Can you work these out from the model? Positions are in its coordinate system, mm. Face numbers are marked on the shaded views. A direction names the side the tool comes from. Give positions to 0.01 mm unless a question says otherwise; leave off trailing zeros. Order: outer loops, then holes, each group sorted by start corner. A loop starts at its lowest first (then second) coordinate and runs counter-clockwise, first axis right, second up. Notation, with made-up numbers: (-8, 26.25) - (27, 26.25) arc R24 cw to (27, 44.25) - close; hole circle Ø6 at (8, 41). An arc over 180 degrees is marked (long way). One line per question, with ' | ' between items.
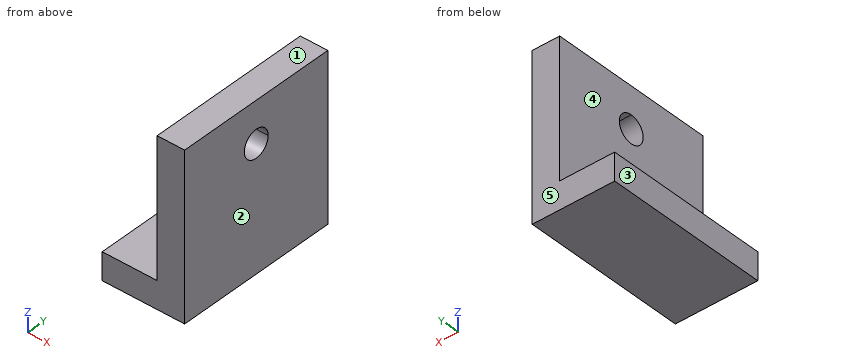
```python
from build123d import *

# Parameters (mm, degrees)
F1_DEPTH = 76.2
F3_DEPTH = 50.8


with BuildPart() as f1:
    # F0 (on Front) → F1 (new body, symmetric)
    with BuildSketch(Plane.XZ):
        Polygon((-76.2, 0), (0, 0), (0, 152.4), (-25.4, 152.4), (-25.4, 25.4), (-76.2, 25.4), align=None)
    extrude(amount=F1_DEPTH, both=True)

    # F2 (on face) → F3 (cut)
    with BuildSketch(Plane.YZ):
        with BuildLine():
            Line((0, 114.3), (0, 127))
            ThreePointArc((0, 127), (-8.980256, 105.319744), (12.7, 114.3))
            Line((12.7, 114.3), (0, 114.3))
        make_face()
        with BuildLine():
            ThreePointArc((12.7, 114.3), (8.980256, 123.280256), (0, 127))
            Line((0, 127), (0, 114.3))
            Line((0, 114.3), (12.7, 114.3))
        make_face()
    extrude(amount=-F3_DEPTH, mode=Mode.SUBTRACT)


solid = f1.part
```
(1) Imagine slicing it at B-B (y = -29). List the corners of the cut face in (x, z) for me, and give its area (3 significant figures).
Answer below:
outline: (-76.2, 0) - (0, 0) - (0, 152.4) - (-25.4, 152.4) - (-25.4, 25.4) - (-76.2, 25.4) - close | area: 5,160 mm^2
(2) On a 3-axis mill with a long thin cutter (end or side, diameter ignored), from which of +Z, -Z, +X, -X, +Y, -Y can I reach the whole of each face in a straight line? I mean the marked faces 4 and 5. Say none if no direction works.
Answer below:
face 4: +Z, -X, +Y, -Y | face 5: +Z, -Z, +X, -X, +Y
(3) Imagine slicing it at A-A (z = 106.5). List the corners of the cut face in (x, y) for me, and give its area (3 significant figures).
Answer below:
outline: (-25.4, -76.2) - (0, -76.2) - (0, -10.02) - (-25.4, -10.02) - close; (-25.4, 10.02) - (0, 10.02) - (0, 76.2) - (-25.4, 76.2) - close | area: 3,360 mm^2
(4) Imagine slicing it at D-D (z = 135.5). List the corners of the cut face in (x, y) for me.
Answer below:
outline: (-25.4, -76.2) - (0, -76.2) - (0, 76.2) - (-25.4, 76.2) - close
(5) Will this pin go through, and if not, where does the flat tip stop? pin 1 (10 mm diameter, centred on x = -45.5, y = -41.5, fed in from +Z).
Answer below:
pin 1: z = 25.4
(6) If we mould it in two halves opening along X, with no side actions, what happens to the marked faces 1, 2 and 3? For each: released by +X, released by -X, zero draft, split by the parting line, or undercut.
Answer below:
face 1: zero draft | face 2: released by +X | face 3: released by -X
(7) If I drill on line 1 (Y direction, x = -11.25, z = 114.3); line 2 (Z direction, x = -10.25, y = 0); line 3 (X direction, y = 66.5, z = 110), over which ranges is the centre line in solid material (lowest first)?
Answer below:
line 1: -76.2 to -12.7, 12.7 to 76.2 | line 2: 0 to 101.6, 127 to 152.4 | line 3: -25.4 to 0
(8) Imagine slicing it at C-C (x = -71). List the corners of the cut face in (y, z) for me.
Answer below:
outline: (-76.2, 0) - (76.2, 0) - (76.2, 25.4) - (-76.2, 25.4) - close
